Design review of the part built by this model. Coordinates are the model's own, in mm. Give positions to 0.01 mm unless a question says otherwise; leave off trailing zeros. Loops run counter-clockwise (first coordinate to the right, second up) from the corner with the lowest first, then second, coordinate; pieces in that order, holes last. Notation, with made-up numbers: (31, 81.25) - (80, 81.25) arc R17 ccw to (80, 99.25) - close; hole circle Ø2 at (70, -19.5). An arc over 180 degrees is marked (long way). Put each result on its own line as item: value. Start each with the question number.
```python
from build123d import *

# Parameters (mm, degrees)
BOX_W     = 32
BOX_H     = 32
BOX_DEPTH = 6


with BuildPart() as esfera003:
    # Sphere003 → Sphere003 (revolve)
    with BuildSketch(Plane(origin=(10, 0, 0), x_dir=(1, 0, 0), z_dir=(0, -1, 0))):
        with BuildLine():
            ThreePointArc((0, -5), (5, 0), (0, 5))
            Line((0, 5), (0, -5))
        make_face()
    revolve(axis=Axis((10, 0, 0), (0, 0, 1)))


with BuildPart() as esfera002:
    # Sphere002 → Sphere002 (revolve)
    with BuildSketch(Plane.XZ.offset(-20)):
        with BuildLine():
            ThreePointArc((0, -5), (5, 0), (0, 5))
            Line((0, 5), (0, -5))
        make_face()
    revolve(axis=Axis((0, 20, 0), (0, 0, 1)))


with BuildPart() as esfera:
    # Sphere → Sphere (revolve)
    with BuildSketch(Plane.XZ):
        with BuildLine():
            ThreePointArc((0, -5), (5, 0), (0, 5))
            Line((0, 5), (0, -5))
        make_face()
    revolve(axis=Axis((0, 0, 0), (0, 0, 1)))


with BuildPart() as esfera001:
    # Sphere001 → Sphere001 (revolve)
    with BuildSketch(Plane.XZ.offset(-10)):
        with BuildLine():
            ThreePointArc((0, -5), (5, 0), (0, 5))
            Line((0, 5), (0, -5))
        make_face()
    revolve(axis=Axis((0, 10, 0), (0, 0, 1)))


with BuildPart() as esfera004:
    # Sphere004 → Sphere004 (revolve)
    with BuildSketch(Plane(origin=(10, 10, 0), x_dir=(1, 0, 0), z_dir=(0, -1, 0))):
        with BuildLine():
            ThreePointArc((0, -5), (5, 0), (0, 5))
            Line((0, 5), (0, -5))
        make_face()
    revolve(axis=Axis((10, 10, 0), (0, 0, 1)))


with BuildPart() as esfera007:
    # Sphere007 → Sphere007 (revolve)
    with BuildSketch(Plane(origin=(20, 10, 0), x_dir=(1, 0, 0), z_dir=(0, -1, 0))):
        with BuildLine():
            ThreePointArc((0, -5), (5, 0), (0, 5))
            Line((0, 5), (0, -5))
        make_face()
    revolve(axis=Axis((20, 10, 0), (0, 0, 1)))


with BuildPart() as esfera005:
    # Sphere005 → Sphere005 (revolve)
    with BuildSketch(Plane(origin=(10, 20, 0), x_dir=(1, 0, 0), z_dir=(0, -1, 0))):
        with BuildLine():
            ThreePointArc((0, -5), (5, 0), (0, 5))
            Line((0, 5), (0, -5))
        make_face()
    revolve(axis=Axis((10, 20, 0), (0, 0, 1)))


with BuildPart() as esfera006:
    # Sphere006 → Sphere006 (revolve)
    with BuildSketch(Plane(origin=(20, 0, 0), x_dir=(1, 0, 0), z_dir=(0, -1, 0))):
        with BuildLine():
            ThreePointArc((0, -5), (5, 0), (0, 5))
            Line((0, 5), (0, -5))
        make_face()
    revolve(axis=Axis((20, 0, 0), (0, 0, 1)))


with BuildPart() as fusion:
    # Sphere008 → Sphere008 (revolve)
    with BuildSketch(Plane(origin=(20, 20, 0), x_dir=(1, 0, 0), z_dir=(0, -1, 0))):
        with BuildLine():
            ThreePointArc((0, -5), (5, 0), (0, 5))
            Line((0, 5), (0, -5))
        make_face()
    revolve(axis=Axis((20, 20, 0), (0, 0, 1)))

    # Fusion: union Esfera003, Esfera002, Esfera, Esfera001, Esfera004, Esfera007, Esfera005, Esfera006
    add(esfera003.part)
    add(esfera002.part)
    add(esfera.part)
    add(esfera001.part)
    add(esfera004.part)
    add(esfera007.part)
    add(esfera005.part)
    add(esfera006.part)


with BuildPart() as fusion_1:
    # Fusion placement: moved
    add(fusion.part.moved(Location((6, 6, 6))))


with BuildPart() as cut:
    # Box → Box (new body)
    with BuildSketch(Plane.XY):
        with Locations((16, 16)):
            Rectangle(BOX_W, BOX_H)
    extrude(amount=BOX_DEPTH)

    # Cut: cut Fusion
    add(fusion_1.part, mode=Mode.SUBTRACT)


solid = cut.part
```
Item 1: Consider section C-C (z = 4.45). Count the separate pieces of the cut face and the enclosed holes in it, plus the area to 3 significant figures.
Item 2: For L1, parallel to Y at x = 7, z = 5.55; L2, parallel to Y at x = 30, z = 4.05; L3, parallel to X at y = 12.5, z = 4.75, list the stretches that pass through material, from the lowest coordinate up. Write a range as from..to.
Item 3: For P1, Ø2, axis at x = 8, y = 26, coming from the +Z side, flat-tipped, find the tip position at first contact; note if it passes through.
Item 4: Consider section A-A (x = 12). State the section outline as (y, z) points, plus the area to 3 significant figures.
Geometry says:
1. separate pieces: 1
1. enclosed holes: 9
1. area: 385 mm2
2. L1: y = 0..1.12, 10.88..11.12, 20.88..21.12, 30.88..32
2. L2: y = 0..3.72, 8.28..13.72, 18.28..23.72, 28.28..32
2. L3: x = 0..2.66, 9.34..12.66, 19.34..22.66, 29.34..32
3. P1: stops at z = 2
4. outline: (0, 0) - (32, 0) - (32, 6) - (29, 6) arc R3 cw to (23, 6) - (19, 6) arc R3 cw to (13, 6) - (9, 6) arc R3 cw to (3, 6) - (0, 6) - close
4. area: 150 mm2
